The model under review builds one solid part; all positions refer to its coordinate system, in mm. A direction names the side the tool comes from. Coordinates: 2 decimals unless noted, no trailing zeros. Loops run counter-clockwise (first coordinate to the right, second up) from the corner with the lowest first, then second, coordinate; pieces in that order, holes last. Notation, with made-up numbers: M -39.75,-20 L -16.75,-20 A19 ccw -16.75,17 Z; hole C 36,14 d11. An arc over 180 degrees is marked long. Use CSV: the item, a comma, the result in double quotes. Start each with the question number.
1. Add section D-D, the plane x = 3. Write out the cut boundary in (y, z).
2. Draft analysis for pull direction X (two halves, no side actions). For faces 4 (the flat face through (8, -10, -15)), 5 (the cylindrical face through (7.19, -22.32, -8.27)), 6 (the cylindrical face through (28.487, -0.493, -3.195)), state which applies: +X half, -X half, draft (parallel to the pull), parting line (faces both ways), or undercut.
3. For L1, parallel to X at y = -0.2, z = -3; L2, parallel to Y at x = 3, z = -8.5; L3, parallel to X at y = -23.5, z = -10.5, list the stretches that pass through material, from the lowest coordinate up.
4. Add section C-C, the plane y = -27.5. Write out the cut boundary in (x, z), then the cut area to 3 significant figures.
5. Tool access review of faces 1 (the flat face through (0, -5, -10)), 2 (the cylindrical face through (2.93, 0.49, -15.5)), 3 (the flat face through (3, 1, -17)): name each direction out of +Z, -Z, +X, -X, +Y, -Y from which nothing blocks a thin tool from reaching the whole face with its end or side.
6. Add section B-B, the plane z = -10. Write out the cut boundary in (x, y), then the cut area to 3 significant figures.
7. Add section A-A, the plane x = 27. Write out the cut boundary in (y, z).
8. Clearance check with flat-ended pins moving along their axes: P1, Ø1.8, axis at x = 27, z = -3, coming from the -Y side; P2, Ø1.5, axis at x = 3, z = -17, coming from the +Y side; P3, Ø8, axis at x = 11.5, y = -23.5, coming from the -Z side. State where each tip first meets the part, or that it passes through.
from build123d import *

# Parameters (mm, degrees)
SKETCH1_W           = 30
SKETCH1_H           = 20
BOSS_EXTRUDE1_DEPTH = 10
SKETCH2_R           = 8
BOSS_EXTRUDE2_DEPTH = 25
SKETCH3_R           = 9.5
BOSS_EXTRUDE3_DEPTH = 3
SKETCH4_R           = 1.5
BOSS_EXTRUDE4_DEPTH = 1
SKETCH5_R           = 1.5
CUT_EXTRUDE1_DEPTH  = 1


with BuildPart() as part:
    # Sketch1 → Boss-Extrude1 (new body)
    with BuildSketch(Plane(origin=(0, 0, 0), x_dir=(1, 0, 0), z_dir=(0, 1, 0))):
        with Locations((15, 10)):
            Rectangle(SKETCH1_W, SKETCH1_H)
    extrude(amount=-BOSS_EXTRUDE1_DEPTH)

    # Sketch2 → Boss-Extrude2 (add)
    with BuildSketch(Plane.XZ.offset(10)):
        with Locations(Location((15, -10, 0), (0, 0, 270))):
            Circle(SKETCH2_R)
    extrude(amount=BOSS_EXTRUDE2_DEPTH)

    # Sketch3 → Boss-Extrude3 (add)
    with BuildSketch(Plane(origin=(0, 0, 0), x_dir=(1, 0, 0), z_dir=(0, 1, 0))):
        with Locations(Location((15, 10, 0), (0, 0, 270))):
            Circle(SKETCH3_R)
    extrude(amount=BOSS_EXTRUDE3_DEPTH)

    # Sketch4 → Boss-Extrude4 (add)
    with BuildSketch(Plane(origin=(0, 0, 0), x_dir=(1, 0, 0), z_dir=(0, 1, 0))):
        with Locations(Location((3, 17, 0), (0, 0, 90))):
            Circle(SKETCH4_R)
    extrude(amount=BOSS_EXTRUDE4_DEPTH)

    # Sketch5 → Cut-Extrude1 (cut)
    with BuildSketch(Plane(origin=(0, 0, 0), x_dir=(1, 0, 0), z_dir=(0, 1, 0))):
        with Locations(Location((27, 3, 0), (0, 0, 270))):
            Circle(SKETCH5_R)
    extrude(amount=-CUT_EXTRUDE1_DEPTH, mode=Mode.SUBTRACT)


solid = part.part
Computed:
1,outline,"M -10,-20 L 0,-20 L 0,-18.5 L 1,-18.5 L 1,-15.5 L 0,-15.5 L 0,0 L -10,0 Z"
2,face 4,"draft"
2,face 5,"parting line"
2,face 6,"undercut"
3,L1,"x = 0 to 25.5, 28.5 to 30"
3,L2,"y = -10 to 0"
3,L3,"x = 7.02 to 22.98"
4,outline,"C 15,-10 d16"
4,area,"201 mm^2"
5,face 1,"+Z, -Z, -X, +Y, -Y"
5,face 2,"+Y"
5,face 3,"+Z, -Z, -X, +Y"
6,outline,"M 0,-10 L 7,-10 L 7,-35 L 23,-35 L 23,-10 L 30,-10 L 30,0 L 24.5,0 L 24.5,3 L 5.5,3 L 5.5,0 L 0,0 Z"
6,area,"757 mm^2"
7,outline,"M -10,-20 L 0,-20 L 0,-4.5 L -1,-4.5 L -1,-1.5 L 0,-1.5 L 0,0 L -10,0 Z"
8,P1,"stops at y = -10"
8,P2,"stops at y = 1"
8,P3,"stops at z = -18"
